The model under review builds one solid part; all positions refer to its coordinate system, in mm. A direction names the side the tool comes from. Round coordinates to 2 decimals unless told otherwise and drop trailing zeros. Write each loop counter-clockwise with the first axis right and the second up, starting at its lowest first coordinate (ties: lowest second). Pieces come first, ordered by that corner, then holes. Notation, with made-up numbers: (46, 12) -> (85, 12) arc R11 cw to (85, 19) -> close; hole circle Ø2 at (66.25, -33). An arc over 180 degrees is marked (long way). Answer in a Markdown table with one row per item. Add a question column.
```python
from build123d import *

# Parameters (mm, degrees)
BOSS_EXTRUDE1_DEPTH = 10
SKETCH3_R           = 0.75
CUT_EXTRUDE1_DEPTH  = 19.317085603
SKETCH4_W           = 3.75
SKETCH4_H           = 1.9
BOSS_EXTRUDE2_DEPTH = 1


with BuildPart() as part:
    # Sketch2 → Boss-Extrude1 (new body)
    with BuildSketch(Plane.XY):
        Polygon((-12.625, 6), (-14.125, 6), (-14.125, 0), (14.125, 0), (14.125, 6), (12.625, 6), (12.625, 1.5), (-12.625, 1.5), align=None)
    extrude(amount=BOSS_EXTRUDE1_DEPTH)

    # Sketch3 → Cut-Extrude1 (cut, through all)
    with BuildSketch(Plane.XY.offset(10)):
        with Locations((-11.25, 1.75)):
            Circle(SKETCH3_R)
        with Locations((-8.75, 1.75)):
            Circle(SKETCH3_R)
        with Locations((-6.25, 1.75)):
            Circle(SKETCH3_R)
        with Locations((-3.75, 1.75)):
            Circle(SKETCH3_R)
        with Locations((-1.25, 1.75)):
            Circle(SKETCH3_R)
        with Locations((1.25, 1.75)):
            Circle(SKETCH3_R)
        with Locations((3.75, 1.75)):
            Circle(SKETCH3_R)
        with Locations((6.25, 1.75)):
            Circle(SKETCH3_R)
        with Locations((8.75, 1.75)):
            Circle(SKETCH3_R)
        with Locations((11.25, 1.75)):
            Circle(SKETCH3_R)
    extrude(amount=-CUT_EXTRUDE1_DEPTH, mode=Mode.SUBTRACT)

    # Sketch4 → Boss-Extrude2 (add)
    with BuildSketch(Plane(origin=(-12.625, 0, 0), x_dir=(0, 0, -1), z_dir=(1, 0, 0))):
        with Locations((-5, 5.05)):
            Rectangle(SKETCH4_W, SKETCH4_H)
    boss_extrude2 = extrude(amount=BOSS_EXTRUDE2_DEPTH)

    # Mirror1: Boss-Extrude2 across plane
    add(boss_extrude2.mirror(Plane.ZY))


solid = part.part
```
1. Tool access review of faces 5 (the flat face through (12, 5, 3.125)), 6 (the flat face through (10, 1.5, 5)), 7 (the flat face through (12.625, 3.8, 4.9)): name each direction out of +Z, -Z, +X, -X, +Y, -Y from which nothing blocks a thin tool from reaching the whole face with its end or side.
2. For L1, parallel to X at y = 3.6, z = 2.75 (3 decimals); L2, parallel to X at y = 4.3, z = 4.75 (3 decimals); L3, parallel to Y at x = 10.25, z = 2.75, list the stretches that pass through material, from the lowest coordinate up.
3. Add section D-D on x = 7.5. Write out the cut boundary in (y, z), plus the area to 3 significant figures.
4. Add section A-A on y = 3.15. Write out the cut boundary in (x, z) (3 decimals), plus the area to 3 significant figures.
5. Mouldability with a two-part tool opening along X and no side actions: class faces 1 (the flat face through (12, 4.1, 5)), 2 (the cylindrical face through (3.7, 1, 5.1)), 3 (the flat face through (0, 0, 5)), 4 (the flat face through (-14.125, 3, 5)) as pulls with the +X half, pulls with the -X half, needs draft (parallel to the pull), parting line crosses it, or undercut.
6. Add section B-B on z = 7.25. Write out the cut boundary in (x, y) (3 decimals).
7. Add section C-C on y = 5. Write out the cut boundary in (x, z) (3 decimals), plus the area to 3 significant figures.
8. Insertion check: pin 1 Ø1.1 at (x, y) = (-12, 5) entering from +Z (3 decimals); pin 2 Ø1.2 at (x, z) = (10, 7.5) entering from +Y. Each pin has a flat end and moves straight along its axis. Give the tip position at first contact, or say it passes through.
Filled in:
| question | item | result |
|---|---|---|
| 1 | face 5 | -Z, +Y |
| 1 | face 6 | +Z, -Z, +Y |
| 1 | face 7 | none |
| 2 | L1 | -14.125 to -12.625, 12.625 to 14.125 |
| 2 | L2 | -14.125 to -11.625, 11.625 to 14.125 |
| 2 | L3 | 0 to 1.5 |
| 3 | outline | (0, 0) -> (1.5, 0) -> (1.5, 10) -> (0, 10) -> close |
| 3 | area | 15.0 mm² |
| 4 | outline | (-14.125, 0) -> (-12.625, 0) -> (-12.625, 10) -> (-14.125, 10) -> close; (12.625, 0) -> (14.125, 0) -> (14.125, 10) -> (12.625, 10) -> close |
| 4 | area | 30.0 mm² |
| 5 | face 1 | undercut |
| 5 | face 2 | undercut |
| 5 | face 3 | needs draft |
| 5 | face 4 | pulls with the -X half |
| 6 | outline | (-14.125, 0) -> (14.125, 0) -> (14.125, 6) -> (12.625, 6) -> (12.625, 1.5) -> (11.957, 1.5) arc R0.75 cw to (10.543, 1.5) -> (9.457, 1.5) arc R0.75 cw to (8.043, 1.5) -> (6.957, 1.5) arc R0.75 cw to (5.543, 1.5) -> (4.457, 1.5) arc R0.75 cw to (3.043, 1.5) -> (1.957, 1.5) arc R0.75 cw to (0.543, 1.5) -> (-0.543, 1.5) arc R0.75 cw to (-1.957, 1.5) -> (-3.043, 1.5) arc R0.75 cw to (-4.457, 1.5) -> (-5.543, 1.5) arc R0.75 cw to (-6.957, 1.5) -> (-8.043, 1.5) arc R0.75 cw to (-9.457, 1.5) -> (-10.543, 1.5) arc R0.75 cw to (-11.957, 1.5) -> (-12.625, 1.5) -> (-12.625, 6) -> (-14.125, 6) -> close |
| 7 | outline | (-14.125, 0) -> (-12.625, 0) -> (-12.625, 3.125) -> (-11.625, 3.125) -> (-11.625, 6.875) -> (-12.625, 6.875) -> (-12.625, 10) -> (-14.125, 10) -> close; (11.625, 3.125) -> (12.625, 3.125) -> (12.625, 0) -> (14.125, 0) -> (14.125, 10) -> (12.625, 10) -> (12.625, 6.875) -> (11.625, 6.875) -> close |
| 7 | area | 37.5 mm² |
| 8 | pin 1 | z = 6.875 |
| 8 | pin 2 | y = 1.5 |
